from build123d import *

# Parameters (mm, degrees)
SKETCH_1_R          = 4
SKETCH_1_R_2        = 1.25
EXTRUDE_1_DEPTH     = 4.5
SKETCH_2_R          = 1
EXTRUDE_2_DEPTH     = 1.9
SKETCH_3_R          = 2.4
CUT_EXTRUDE_1_DEPTH = 3


with BuildPart() as part:
    # 草图1 → 凸台-拉伸1 (new body)
    with BuildSketch(Plane(origin=(0, 0, 0), x_dir=(1, 0, 0), z_dir=(0, 1, 0))):
        Circle(SKETCH_1_R)
        Circle(SKETCH_1_R_2, mode=Mode.SUBTRACT)
    extrude(amount=EXTRUDE_1_DEPTH)

    # 草图2 → 凸台-拉伸2 (add)
    with BuildSketch(Plane(origin=(0, 4.5, 0), x_dir=(1, 0, 0), z_dir=(0, 1, 0))):
        with BuildLine():
            Line((19.197368421, 2.492196964), (0.315789474, 3.987515142))
            ThreePointArc((0.315789474, 3.987515142), (4, 0), (0.315789474, -3.987515142))
            Line((0.315789474, -3.987515142), (19.197368421, -2.492196964))
            ThreePointArc((19.197368421, -2.492196964), (21.5, 0), (19.197368421, 2.492196964))
        make_face()
        with Locations((16, 0)):
            Circle(SKETCH_2_R, mode=Mode.SUBTRACT)
        with Locations((10, 0)):
            Circle(SKETCH_2_R, mode=Mode.SUBTRACT)
        with Locations((13, 0)):
            Circle(SKETCH_2_R, mode=Mode.SUBTRACT)
        with Locations((19, 0)):
            Circle(SKETCH_2_R, mode=Mode.SUBTRACT)
    extrude(amount=-EXTRUDE_2_DEPTH)

    # 草图3 → 切除-拉伸1 (cut)
    with BuildSketch(Plane.XZ):
        Circle(SKETCH_3_R)
    extrude(amount=-CUT_EXTRUDE_1_DEPTH, mode=Mode.SUBTRACT)


solid = part.part
Read the model definition and answer for the solid it produces. Units are mm, in the model's axes. A direction names the side the tool comes from. Round coordinates to 2 decimals unless told otherwise and drop trailing zeros. Write each loop counter-clockwise with the first axis right and the second up, starting at its lowest first coordinate (ties: lowest second). Pieces come first, ordered by that corner, then holes. Notation, with made-up numbers: (20, 72) - (34, 72) arc R16 cw to (34, 78) - close; hole circle Ø9 at (-26, 21.5). An arc over 180 degrees is marked (long way). Use a Markdown table: item, result.
(1) Which of the six approach directions +Z, -Z, +X, -X, +Y, -Y give full straight-line access (tool end or side, diameter ignored) to faces 1 (the cylindrical face through (1.29, 1.479, 2.024)), 2 (the cylindrical face through (21.5, 3.6, 0.1))?
Reported:
| item | result |
|---|---|
| face 1 | -Y |
| face 2 | +X, +Y, -Y |
(2) The part is cut by section B-B (x = 0). Write down the section's boundary in (y, z), then the cut area to 4 significant figures.
Reported:
| item | result |
|---|---|
| outline | (0, -4) - (4.5, -4) - (4.5, -1.25) - (3, -1.25) - (3, -2.4) - (0, -2.4) - close; (0, 2.4) - (3, 2.4) - (3, 1.25) - (4.5, 1.25) - (4.5, 4) - (0, 4) - close |
| area | 17.85 mm2 |
(3) The mould has two halves that part along X. Classify faces 3 (the cylindrical face through (-4, 2, 0)), 4 (the cylindrical face through (-0.27, 3.74, 1.22)), 5 (the flat face through (11, 2.6, 1)), 6 (the flat face through (9.62, 3.56, 3.25)): released by +X, released by -X, zero draft, split by the parting line, or undercut.
Reported:
| item | result |
|---|---|
| face 3 | split by the parting line |
| face 4 | undercut |
| face 5 | zero draft |
| face 6 | released by +X |
(4) The part is cut by section A-A (z = 0). State how many separate pieces and enclosed holes the cut face has, then the cut area to 3 significant figures.
Reported:
| item | result |
|---|---|
| separate pieces | 6 |
| enclosed holes | 0 |
| area | 35.9 mm2 |
(5) Each of these flat-tipped pins is pushed along its axis until it touches: pin 1 Ø3 at (x, z) = (13, 0) entering from -Y; pin 2 Ø4 at (x, z) = (0, 0) entering from +Y; pin 3 Ø1.5 at (x, y) = (12, 3) entering from -Z; pin 4 Ø2 at (y, z) = (2, 2) entering from +X. Where does it stop, or does it pass through?
Reported:
| item | result |
|---|---|
| pin 1 | y = 2.6 |
| pin 2 | y = 4.5 |
| pin 3 | z = -3.12 |
| pin 4 | x = 21.19 |
(6) The part is cut by section C-C (y = 3.9). Write down the section's boundary in (x, z), then the cut area to 3 significant figures.
Reported:
| item | result |
|---|---|
| outline | (0.32, -3.99) - (19.2, -2.49) arc R2.5 ccw to (19.2, 2.49) - (0.32, 3.99) arc R4 ccw (long way) to start; hole circle Ø2.5 at (0, 0); hole circle Ø2 at (10, 0); hole circle Ø2 at (13, 0); hole circle Ø2 at (16, 0); hole circle Ø2 at (19, 0) |
| area | 141 mm2 |
(7) Straight lines are drawn through the part: line 1 along X through (y, z) = (3.75, 0); line 2 along Z through (x, y) = (0, 3.8); line 3 along Y through (x, z) = (5, -0.25). For each, find the intervals that lie inside material, in ascending order. Write a range as [from, to].
Reported:
| item | result |
|---|---|
| line 1 | [-4, -1.25], [1.25, 9], [11, 12], [14, 15], [17, 18], [20, 21.5] |
| line 2 | [-4, -1.25], [1.25, 4] |
| line 3 | [2.6, 4.5] |
(8) The part is cut by section D-D (z = 2). Write down the section's boundary in (x, y).
Reported:
| item | result |
|---|---|
| outline | (-3.46, 0) - (-1.33, 0) - (-1.33, 3) - (1.33, 3) - (1.33, 0) - (3.46, 0) - (3.46, 2.6) - (20.5, 2.6) - (20.5, 4.5) - (-3.46, 4.5) - close |
